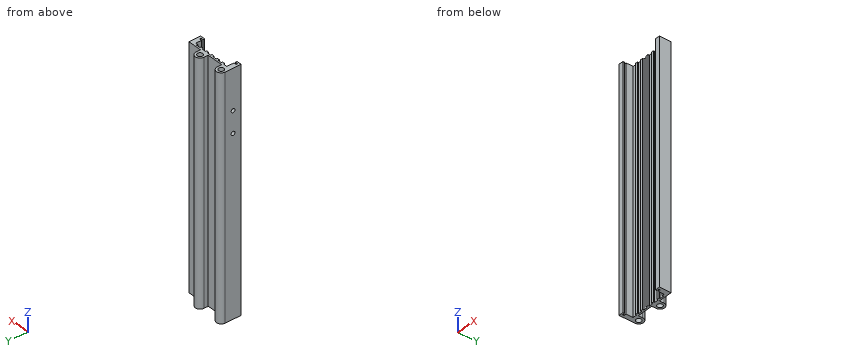
from build123d import *

# Parameters (mm, degrees)
SKETCH1_R           = 2.159
BOSS_EXTRUDE1_DEPTH = 195.58
SKETCH2_R           = 1.5875
CUT_EXTRUDE1_DEPTH  = 2.54


with BuildPart() as part:
    # Sketch1 → Boss-Extrude1 (new body)
    with BuildSketch(Plane.XY):
        with BuildLine():
            Line((0, 0), (-4.064, 0))
            Line((-4.064, 0), (-4.064, 9.652))
            Line((-4.064, 9.652), (-4.064, 13.2588))
            ThreePointArc((-4.064, 13.2588), (-0.254, 17.0688), (3.556, 13.2588))
            Line((3.556, 13.2588), (3.556, 9.652))
            Line((3.556, 9.652), (16.891, 9.652))
            Line((16.891, 9.652), (16.891, 13.2588))
            ThreePointArc((16.891, 13.2588), (20.701, 17.0688), (24.511, 13.2588))
            Line((24.511, 13.2588), (24.511, 9.652))
            Line((24.511, 9.652), (36.068, 9.652))
            Line((36.068, 9.652), (36.068, 0))
            Line((36.068, 0), (32.004, 0))
            Line((32.004, 0), (32.004, 1.27))
            Line((32.004, 1.27), (34.036, 1.27))
            Line((34.036, 1.27), (34.036, 2.54))
            Line((34.036, 2.54), (32.004, 2.54))
            Line((32.004, 2.54), (32.004, 7.366))
            Line((32.004, 7.366), (29.972, 7.366))
            Line((29.972, 7.366), (29.972, 8.382))
            Line((29.972, 8.382), (26.67, 8.382))
            Line((26.67, 8.382), (26.67, 7.366))
            Line((26.67, 7.366), (24.638, 7.366))
            Line((24.638, 7.366), (24.638, 8.382))
            Line((24.638, 8.382), (21.336, 8.382))
            Line((21.336, 8.382), (21.336, 7.366))
            Line((21.336, 7.366), (19.304, 7.366))
            Line((19.304, 7.366), (19.304, 8.382))
            Line((19.304, 8.382), (16.002, 8.382))
            Line((16.002, 8.382), (16.002, 7.366))
            Line((16.002, 7.366), (13.97, 7.366))
            Line((13.97, 7.366), (13.97, 8.382))
            Line((13.97, 8.382), (10.668, 8.382))
            Line((10.668, 8.382), (10.668, 7.366))
            Line((10.668, 7.366), (8.636, 7.366))
            Line((8.636, 7.366), (8.636, 8.382))
            Line((8.636, 8.382), (5.334, 8.382))
            Line((5.334, 8.382), (5.334, 7.366))
            Line((5.334, 7.366), (3.302, 7.366))
            Line((3.302, 7.366), (3.302, 8.382))
            Line((3.302, 8.382), (0, 8.382))
            Line((0, 8.382), (0, 2.54))
            Line((0, 2.54), (-2.032, 2.54))
            Line((-2.032, 2.54), (-2.032, 1.27))
            Line((-2.032, 1.27), (0, 1.27))
            Line((0, 1.27), (0, 0))
        make_face()
        with Locations((-0.254, 13.2588)):
            Circle(SKETCH1_R, mode=Mode.SUBTRACT)
        with Locations((20.701, 13.2588)):
            Circle(SKETCH1_R, mode=Mode.SUBTRACT)
    extrude(amount=-BOSS_EXTRUDE1_DEPTH)

    # Sketch2 → Cut-Extrude1 (cut)
    with BuildSketch(Plane.ZY.offset(4.064)):
        with Locations((-33.02, 6.6294)):
            Circle(SKETCH2_R)
        with Locations((-50.8, 6.6294)):
            Circle(SKETCH2_R)
    extrude(amount=-CUT_EXTRUDE1_DEPTH, mode=Mode.SUBTRACT)


solid = part.part
Verification items for the finished model (mm, model axes). Coordinates: 2 decimals unless noted, no trailing zeros. Loops run counter-clockwise (first coordinate to the right, second up) from the corner with the lowest first, then second, coordinate; pieces in that order, holes last. Notation, with made-up numbers: M 33.5,22.25 L 50.5,22.25 A27 ccw 50.5,57.25 Z; hole C 43.5,-34.5 d3. An arc over 180 degrees is marked long. One line per item, written item: value.
1. Gauge pin test, flat ends, axial feed: P1, Ø1.6, axis at x = 26, z = -79, coming from the -Y side; P2, Ø4, axis at x = 13, y = 12, coming from the +Z side; P3, Ø14.5, axis at x = 11.5, z = -123.5, coming from the +Y side; P4, Ø2.5, axis at x = 1.5, z = -112, coming from the -Y side. Record the tip position at first contact, or that the pin passes through.
Answers follow:
P1: y = 7.37
P2: through
P3: y = 16.53
P4: y = 8.38
2. Material ranges on line 1 along X through (y, z) = (5.25, -104.5); line 2 along X through (y, z) = (12.5, -141.5); line 3 along Y through (x, z) = (32.5, -93), recorded low to high. Write a range as from..to.
Answers follow:
line 1: -4.06..0, 32..36.07
line 2: -4.06..-2.28, 1.77..3.56, 16.89..18.68, 22.72..24.51
line 3: 0..1.27, 2.54..9.65
3. Section check B-B on x = 7. Record the cut outline in (y, z).
Answers follow:
outline: M 8.38,-195.58 L 9.65,-195.58 L 9.65,0 L 8.38,0 Z
4. Section check A-A on z = -38.5. Give the number of separate pieces and of enclosed holes in the cut face, plus the area to 3 significant figures.
Answers follow:
separate pieces: 1
enclosed holes: 2
area: 198 mm^2
